Geometry check sheet. Reference: the model listing, model coordinates, mm. A direction names the side the tool comes from. Give positions to 0.01 mm unless a question says otherwise; leave off trailing zeros. Loops run counter-clockwise (first coordinate to the right, second up) from the corner with the lowest first, then second, coordinate; pieces in that order, holes last. Notation, with made-up numbers: (7, 77.5) -> (51, 77.5) arc R22 cw to (51, 106.5) -> close; hole circle Ø7 at (82.25, -21). An arc over 180 degrees is marked (long way). Answer as a JSON object with one key per item and string values.
from build123d import *

# Parameters (mm, degrees)
SKETCH1_W           = 140
SKETCH1_H           = 100
BOSS_EXTRUDE1_DEPTH = 3
SKETCH2_R           = 1
CUT_EXTRUDE1_DEPTH  = 3
CUT_EXTRUDE2_REACH  = 88.076
SKETCH3_R           = 1
CUT_EXTRUDE3_REACH  = 88.076
SKETCH4_R           = 0.75
SKETCH4_W           = 30
SKETCH4_H           = 30
FILLET1_R           = 3
CUT_EXTRUDE4_REACH  = 88.076
SKETCH5_W           = 5
SKETCH5_H           = 20
CUT_EXTRUDE5_REACH  = 88.076
SKETCH6_W           = 3
SKETCH6_H           = 6


with BuildPart() as part:
    # Sketch1 → Boss-Extrude1 (new body)
    with BuildSketch(Plane.XY):
        Rectangle(SKETCH1_W, SKETCH1_H)
    extrude(amount=BOSS_EXTRUDE1_DEPTH)

    # Sketch2 → Cut-Extrude1 (cut)
    with BuildSketch(Plane.XY.offset(3)):
        with Locations((30, 38.5)):
            Circle(SKETCH2_R)
        with Locations((-30, 38.5)):
            Circle(SKETCH2_R)
        with Locations((30, -38.5)):
            Circle(SKETCH2_R)
        with Locations((-30, -38.5)):
            Circle(SKETCH2_R)
    extrude(amount=-CUT_EXTRUDE1_DEPTH, mode=Mode.SUBTRACT)

    # Sketch3 → Cut-Extrude2 (cut, up to next)
    with BuildSketch(Plane.XY.offset(3), mode=Mode.PRIVATE) as cut_extrude2_sk1:
        with Locations((34, 32)):
            Circle(SKETCH3_R)
    cut_extrude2_tool1 = extrude(cut_extrude2_sk1.sketch, amount=-CUT_EXTRUDE2_REACH, mode=Mode.PRIVATE) & part.part
    # Sketch3 → Cut-Extrude2 (cut, up to next)
    with BuildSketch(Plane.XY.offset(3), mode=Mode.PRIVATE) as cut_extrude2_sk2:
        with Locations((34, -32)):
            Circle(SKETCH3_R)
    cut_extrude2_tool2 = extrude(cut_extrude2_sk2.sketch, amount=-CUT_EXTRUDE2_REACH, mode=Mode.PRIVATE) & part.part
    # Sketch3 → Cut-Extrude2 (cut, up to next)
    with BuildSketch(Plane.XY.offset(3), mode=Mode.PRIVATE) as cut_extrude2_sk3:
        with Locations((-34, 32)):
            Circle(SKETCH3_R)
    cut_extrude2_tool3 = extrude(cut_extrude2_sk3.sketch, amount=-CUT_EXTRUDE2_REACH, mode=Mode.PRIVATE) & part.part
    # Sketch3 → Cut-Extrude2 (cut, up to next)
    with BuildSketch(Plane.XY.offset(3), mode=Mode.PRIVATE) as cut_extrude2_sk4:
        with Locations((-34, -32)):
            Circle(SKETCH3_R)
    cut_extrude2_tool4 = extrude(cut_extrude2_sk4.sketch, amount=-CUT_EXTRUDE2_REACH, mode=Mode.PRIVATE) & part.part
    add(cut_extrude2_tool1.solids().sort_by_distance((34, 32, 3))[0], mode=Mode.SUBTRACT)
    add(cut_extrude2_tool2.solids().sort_by_distance((34, -32, 3))[0], mode=Mode.SUBTRACT)
    add(cut_extrude2_tool3.solids().sort_by_distance((-34, 32, 3))[0], mode=Mode.SUBTRACT)
    add(cut_extrude2_tool4.solids().sort_by_distance((-34, -32, 3))[0], mode=Mode.SUBTRACT)

    # Sketch4 → Cut-Extrude3 (cut, up to next)
    with BuildSketch(Plane.XY.offset(3), mode=Mode.PRIVATE) as cut_extrude3_sk1:
        with Locations((-65, 15)):
            Circle(SKETCH4_R)
    cut_extrude3_tool1 = extrude(cut_extrude3_sk1.sketch, amount=-CUT_EXTRUDE3_REACH, mode=Mode.PRIVATE) & part.part
    # Sketch4 → Cut-Extrude3 (cut, up to next)
    with BuildSketch(Plane.XY.offset(3), mode=Mode.PRIVATE) as cut_extrude3_sk2:
        with Locations((-65, -15)):
            Circle(SKETCH4_R)
    cut_extrude3_tool2 = extrude(cut_extrude3_sk2.sketch, amount=-CUT_EXTRUDE3_REACH, mode=Mode.PRIVATE) & part.part
    # Sketch4 → Cut-Extrude3 (cut, up to next)
    with BuildSketch(Plane.XY.offset(3), mode=Mode.PRIVATE) as cut_extrude3_sk3:
        Rectangle(SKETCH4_W, SKETCH4_H)
    cut_extrude3_tool3 = extrude(cut_extrude3_sk3.sketch, amount=-CUT_EXTRUDE3_REACH, mode=Mode.PRIVATE) & part.part
    add(cut_extrude3_tool1.solids().sort_by_distance((-65, 15, 3))[0], mode=Mode.SUBTRACT)
    add(cut_extrude3_tool2.solids().sort_by_distance((-65, -15, 3))[0], mode=Mode.SUBTRACT)
    add(cut_extrude3_tool3.solids().sort_by_distance((0, 0, 3))[0], mode=Mode.SUBTRACT)

    # Fillet1
    fillet1_edges = [part.edges().sort_by_distance(p)[0] for p in [
        (70, -50, 1.5),
        (-70, -50, 1.5),
        (-70, 50, 1.5),
        (70, 50, 1.5),
    ]]
    fillet(fillet1_edges, radius=FILLET1_R)

    # Sketch5 → Cut-Extrude4 (cut, up to next)
    with BuildSketch(Plane.XY.offset(3), mode=Mode.PRIVATE) as cut_extrude4_sk1:
        with Locations((-50, 0)):
            Rectangle(SKETCH5_W, SKETCH5_H)
    cut_extrude4_tool1 = extrude(cut_extrude4_sk1.sketch, amount=-CUT_EXTRUDE4_REACH, mode=Mode.PRIVATE) & part.part
    add(cut_extrude4_tool1.solids().sort_by_distance((-50, 0, 3))[0], mode=Mode.SUBTRACT)

    # Sketch6 → Cut-Extrude5 (cut, up to next)
    with BuildSketch(Plane.XY.offset(3), mode=Mode.PRIVATE) as cut_extrude5_sk1:
        with Locations((-62, 0)):
            Rectangle(SKETCH6_W, SKETCH6_H)
    cut_extrude5_tool1 = extrude(cut_extrude5_sk1.sketch, amount=-CUT_EXTRUDE5_REACH, mode=Mode.PRIVATE) & part.part
    add(cut_extrude5_tool1.solids().sort_by_distance((-62, 0, 3))[0], mode=Mode.SUBTRACT)


solid = part.part
1) Section check A-A on y = -7. Record the cut outline in (x, z), plus the area to 3 significant figures.
Geometry check:
{"outline": "(-70, 0) -> (-52.5, 0) -> (-52.5, 3) -> (-70, 3) -> close; (-47.5, 0) -> (-15, 0) -> (-15, 3) -> (-47.5, 3) -> close; (15, 0) -> (70, 0) -> (70, 3) -> (15, 3) -> close", "area": "315 mm2"}
2) Draft check along X on faces 3 (the face through (69.1, -49.14, 1.52)), 4 (the face through (-17, 1, 0)), 5 (the face through (0, 15, 2)). Enter one of: pulls with the +X half, pulls with the -X half, needs draft (parallel to the pull), parting line crosses it, or undercut.
Geometry check:
{"face 3": "pulls with the +X half", "face 4": "needs draft", "face 5": "undercut"}
3) Section check B-B on z = 1.1. Count the separate pieces of the cut face and the enclosed holes in it, plus the area to 3 significant figures.
Geometry check:
{"separate pieces": "1", "enclosed holes": "13", "area": "12,900 mm2"}
4) Section check C-C on x = -11.5. Record the cut outline in (y, z).
Geometry check:
{"outline": "(-50, 0) -> (-15, 0) -> (-15, 3) -> (-50, 3) -> close; (15, 0) -> (50, 0) -> (50, 3) -> (15, 3) -> close"}
5) Depth check by flat-ended pin: P1, Ø1.6, axis at x = -30, y = 38.5, coming from the -Z side. Enter the tip coordinate at first touch or a pass-through.
Geometry check:
{"P1": "passes through"}
6) Material ranges on line 1 along Y through (x, z) = (30, 0.85); line 2 along Y through (x, z) = (-65, 2.1); line 3 along Y through (x, z) = (-8.5, 1.95), recorded low to high. Write a range as from..to.
Geometry check:
{"line 1": "y = -50..-39.5, -37.5..37.5, 39.5..50", "line 2": "y = -50..-15.75, -14.25..14.25, 15.75..50", "line 3": "y = -50..-15, 15..50"}
7) Tool access check on faces 1 (the face through (-62, 3, 2)), 2 (the face through (70, -1, 1)). Record the directions out of +Z, -Z, +X, -X, +Y, -Y that give a thin tool (end or side, any length) a straight path to the whole face; none if there is none.
Geometry check:
{"face 1": "+Z, -Z", "face 2": "+Z, -Z, +X, +Y, -Y"}
